Work out the finished part from the listing and answer in its coordinate system (mm). Face numbers are marked on the shaded views. Coordinates: 2 decimals unless noted, no trailing zeros. Order: outer loops, then holes, each group sorted by start corner. A loop starts at its lowest first (then second) coordinate and runs counter-clockwise, first axis right, second up. Notation, with made-up numbers: (87.5, 35.25) -> (116.5, 35.25) arc R11 cw to (116.5, 47.25) -> close; hole circle Ø8 at (-4, 57.5). An arc over 180 degrees is marked (long way). Write item = value, one per line. Start each with the question number.
Q1. The part is cut by section A-A, the plane z = -1.3. Determine the outline of the cut face in (x, y), plus the area to 3 significant figures.
Q2. Straight lines are drawn through the part: L1, parallel to X at y = -0.4, z = -2.2; L2, parallel to Y at x = 3.5, z = -0.4; L3, parallel to Y at x = 8.25, z = -3.6. For each, find the intervals that lie inside material, in ascending order. Write a range as from..to.
Q3. Flat-ended cylindrical pins translate along their axes: pin 1 (1.2 mm diameter, centred on x = -0.5, z = -2.5, fed in from -Y); pin 2 (0.6 mm diameter, centred on y = -0.5, z = -4, fed in from -X). Find the tip coordinate at first contact, or state that the pin passes through.
Q4. For a pull along Z with two mould halves and no side action, classify the marked faces 1, 2 and 3 as +Z half, -Z half, draft (parallel to the pull), parting line (faces both ways), or undercut.
Q5. The part is cut by section C-C, the plane y = -0.4. Count the separate pieces of the cut face and the enclosed holes in it, plus the area to 3 significant figures.
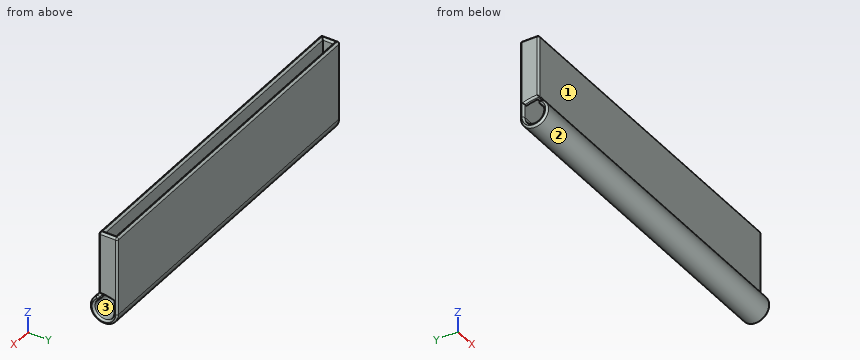
```python
from build123d import *

# Parameters (mm, degrees)
BOSS_EXTRUDE1_DEPTH             = 8.75
BOSS_EXTRUDE2_DEPTH             = 0.2
BOSS_EXTRUDE3_REACH             = 12.005
SKETCH4_W                       = 3.173679441
SKETCH4_H                       = 0.2
BOSS_EXTRUDE3_DIRECTION_2_REACH = 12.005
FILLET1_R                       = 0.09


with BuildPart() as part:
    # Sketch2 → Boss-Extrude1 (new, symmetric)
    with BuildSketch(Plane(origin=(0, 0, 0), x_dir=(0, 0, -1), z_dir=(1, 0, 0))):
        with BuildLine():
            Line((0, 0), (4, 0))
            ThreePointArc((4, 0), (4.425963639, -0.761830056), (3.553879666, -0.725780087))
            Line((3.553879666, -0.725780087), (3.375431533, -0.816092122))
            ThreePointArc((3.375431533, -0.816092122), (4.596349095, -0.866562078), (4, 0.2))
            Line((4, 0.2), (0, 0.2))
            Line((0, 0.2), (0, 0))
        make_face()
    extrude(amount=BOSS_EXTRUDE1_DEPTH, both=True)

    # Sketch3 → Boss-Extrude2 (add)
    with BuildSketch(Plane(origin=(8.75, 0, 0), x_dir=(0, 0, -1), z_dir=(1, 0, 0))):
        with BuildLine():
            Line((0, 0), (0, -0.749873542))
            Line((0, -0.749873542), (3.199706895, -0.749873542))
            ThreePointArc((3.199706895, -0.749873542), (3.230171613, -0.370080622), (3.320786706, 0))
            Line((3.320786706, 0), (0, 0))
        make_face()
    boss_extrude2 = extrude(amount=-BOSS_EXTRUDE2_DEPTH)

    # Mirror1: Boss-Extrude2 across plane
    add(boss_extrude2.mirror(Plane(origin=(0, 0, 0), x_dir=(0, 0, 1), z_dir=(1, 0, 0))))

    # Boss-Extrude3: up to this face of the body (flat: up to its plane)
    boss_extrude3_end = Plane(part.part.faces().sort_by_distance((8.55, -0.372613624, -1.620023342))[0])
    # Sketch4 → Boss-Extrude3 (add, up to the picked face)
    with BuildSketch(Plane(origin=(0, 0, 0), x_dir=(0, 0, -1), z_dir=(1, 0, 0)), mode=Mode.PRIVATE) as boss_extrude3_sk1:
        with Locations((1.58683972, -0.649873542)):
            Rectangle(SKETCH4_W, SKETCH4_H)
    boss_extrude3_tool1 = split(extrude(boss_extrude3_sk1.sketch, amount=BOSS_EXTRUDE3_REACH, mode=Mode.PRIVATE), bisect_by=boss_extrude3_end, keep=Keep.BOTH, mode=Mode.PRIVATE)
    add(boss_extrude3_tool1.solids().sort_by(Axis((0, -0.649874, -1.58684), (1, 0, 0)))[0])

    # Boss-Extrude3 direction 2: up to this face of the body (flat: up to its plane)
    boss_extrude3_direction_2_end = Plane(part.part.faces().sort_by_distance((-8.55, -0.372613624, -1.620023342))[0])
    # Sketch4 → Boss-Extrude3 direction 2 (add, up to the picked face)
    with BuildSketch(Plane(origin=(0, 0, 0), x_dir=(0, 0, -1), z_dir=(1, 0, 0)), mode=Mode.PRIVATE) as boss_extrude3_direction_2_sk1:
        with Locations((1.58683972, -0.649873542)):
            Rectangle(SKETCH4_W, SKETCH4_H)
    boss_extrude3_direction_2_tool1 = split(extrude(boss_extrude3_direction_2_sk1.sketch, amount=-BOSS_EXTRUDE3_DIRECTION_2_REACH, mode=Mode.PRIVATE), bisect_by=boss_extrude3_direction_2_end, keep=Keep.BOTH, mode=Mode.PRIVATE)
    add(boss_extrude3_direction_2_tool1.solids().sort_by(Axis((0, -0.649874, -1.58684), (-1, 0, 0)))[0])

    # Fillet1
    fillet1_edges = [part.edges().sort_by_distance(p)[0] for p in [
        (0, 0.2, 0),
        (0, -0.816092122, -3.375431533),
        (0, -0.725780087, -3.553879666),
        (8.75, -0.761830056, -4.425963639),
        (8.75, -0.770936105, -3.4646556),
        (8.75, 0, -3.660393353),
        (0, 0, 0),
        (8.75, -0.866562078, -4.596349095),
        (8.55, -0.274936771, 0),
        (0, -0.749873542, 0),
        (8.75, -0.749873542, -1.599853447),
        (8.75, -0.370080622, -3.230171613),
        (8.75, 0.2, -2),
        (-8.75, 0, -3.660393353),
        (-8.75, -0.749873542, -1.599853447),
        (-8.75, -0.370080622, -3.230171613),
        (-8.55, -0.274936771, 0),
        (0, -0.549873542, 0),
        (8.75, -0.274936771, 0),
        (-8.75, 0.2, -2),
        (-8.75, -0.866562078, -4.596349095),
        (-8.75, -0.770936105, -3.4646556),
        (-8.75, -0.761830056, -4.425963639),
        (-8.75, -0.274936771, 0),
    ]]
    fillet(fillet1_edges, radius=FILLET1_R)


solid = part.part
```
Model answer:
q1.outline = (-8.75, -0.66) arc R0.09 ccw to (-8.66, -0.75) -> (8.66, -0.75) arc R0.09 ccw to (8.75, -0.66) -> (8.75, 0.11) arc R0.09 ccw to (8.66, 0.2) -> (-8.66, 0.2) arc R0.09 ccw to (-8.75, 0.11) -> close; hole (-8.55, -0.55) -> (8.55, -0.55) -> (8.55, 0) -> (-8.55, 0) -> close
q1.area = 7.21 mm2
q2.L1 = -8.75..-8.55, 8.55..8.75
q2.L2 = -0.75..-0.55, 0..0.2
q2.L3 = -1.07..-0.8, 0..0.2
q3.pin_1 = -0.75
q3.pin_2 = through
q4.face_1 = draft
q4.face_2 = parting line
q4.face_3 = undercut
q5.separate_pieces = 3
q5.enclosed_holes = 0
q5.area = 4.82 mm2
